from build123d import *

# Parameters (mm, degrees)
SKETCH_1_W          = 50
SKETCH_1_H          = 22
SKETCH_1_R          = 1.05
EXTRUDE_1_DEPTH     = 2
SKETCH_2_W          = 25
SKETCH_2_H          = 2
EXTRUDE_2_DEPTH     = 20
SKETCH_3_R          = 1.65
CUT_EXTRUDE_1_DEPTH = 30
SKETCH_4_W          = 35
SKETCH_4_H          = 15
CUT_EXTRUDE_2_DEPTH = 30


with BuildPart() as part:
    # 草图1 → 凸台-拉伸1 (new body)
    with BuildSketch(Plane(origin=(0, 0, 0), x_dir=(1, 0, 0), z_dir=(0, 1, 0))):
        Rectangle(SKETCH_1_W, SKETCH_1_H)
        with Locations(Location((-21.41, 8.87, 0), (0, 0, 270))):
            Circle(SKETCH_1_R, mode=Mode.SUBTRACT)
        with Locations(Location((-21.41, -8.87, 0), (0, 0, 90))):
            Circle(SKETCH_1_R, mode=Mode.SUBTRACT)
        with Locations(Location((21.41, -8.87, 0), (0, 0, 270))):
            Circle(SKETCH_1_R, mode=Mode.SUBTRACT)
        with Locations(Location((21.41, 8.87, 0), (0, 0, 90))):
            Circle(SKETCH_1_R, mode=Mode.SUBTRACT)
    extrude(amount=EXTRUDE_1_DEPTH)

    # 草图2 → 凸台-拉伸2 (add)
    with BuildSketch(Plane(origin=(0, 2, 0), x_dir=(1, 0, 0), z_dir=(0, 1, 0))):
        Rectangle(SKETCH_2_W, SKETCH_2_H)
    extrude(amount=EXTRUDE_2_DEPTH)

    # 草图3 → 切除-拉伸1 (cut)
    with BuildSketch(Plane.XY.offset(1)):
        with Locations((-5, 22)):
            Circle(SKETCH_3_R)
        with Locations((-5, 12)):
            Circle(SKETCH_3_R)
        with Locations((5, 12)):
            Circle(SKETCH_3_R)
        with Locations((5, 22)):
            Circle(SKETCH_3_R)
    extrude(amount=-CUT_EXTRUDE_1_DEPTH, mode=Mode.SUBTRACT)

    # 草图4 → 切除-拉伸2 (cut)
    with BuildSketch(Plane(origin=(0, 2, 0), x_dir=(1, 0, 0), z_dir=(0, 1, 0))):
        with Locations((0, -11)):
            Rectangle(SKETCH_4_W, SKETCH_4_H)
        with Locations((0, 11)):
            Rectangle(SKETCH_4_W, SKETCH_4_H)
    extrude(amount=-CUT_EXTRUDE_2_DEPTH, mode=Mode.SUBTRACT)


solid = part.part
Work out the finished part from the listing and answer in its coordinate system (mm). A direction names the side the tool comes from. Give positions to 0.01 mm unless a question says otherwise; leave off trailing zeros. Order: outer loops, then holes, each group sorted by start corner. A loop starts at its lowest first (then second) coordinate and runs counter-clockwise, first axis right, second up. Notation, with made-up numbers: (40.25, 28) - (94.25, 28) arc R25 ccw to (94.25, 51) - close; hole circle Ø11 at (-4, -38.75). An arc over 180 degrees is marked (long way). Answer as CSV lines item,"result". Start each with the question number.
Q1. Find the intervals of material crossed by L1, parallel to X at y = 0.95, z = -8.87; L2, parallel to Y at x = -5, z = -0.15; L3, parallel to Z at x = 1.5, y = 21.25, in increasing order. Write a range as [from, to].
Q2. The mould has two halves that part along Y. Classify faces 4 (the face through (-6.31, 11, 0.01)), 5 (the face through (10, 22, 0)), 6 (the face through (-25, 1, 0)): +Y half, -Y half, draft (parallel to the pull), parting line (faces both ways), or undercut.
Q3. For faces 1 (the face through (-17.5, 1, -7)), 2 (the face through (-17.5, 1, 7)), 3 (the face through (0, 12, 1)), determine the directions among +Z, -Z, +X, -X, +Y, -Y from which every point of the face is accessible in a straight line to the end or side of a thin tool.
Q4. The part is cut by section D-D (y = 1.5). Write down the section's boundary in (x, z).
Q5. The part is cut by section A-A (z = -8.87). Write down the section's boundary in (x, y), then the cut area to 3 significant figures.
Q6. The part is cut by section B-B (y = 12). Write down the section's boundary in (x, z), then the cut area to 3 significant figures.
Q7. Given pin 1 Ø3 at (x, y) = (9, 4.5) entering from -Z; pin 2 Ø8 at (x, y) = (-3, 18.5) entering from +Z; pin 3 Ø3 at (y, z) = (16, 1) entering from +X, each flat-ended and moving along its own axis, determine where each tip first touches the part or whether it passes through.
Q8. The part is cut by section C-C (x = 21.41). Write down the section's boundary in (y, z), then the cut area to 3 significant figures.
Check result:
1,L1,"x = [-25, -22.46], [-20.36, -17.5], [17.5, 20.36], [22.46, 25]"
1,L2,"y = [0, 10.35], [13.65, 20.35]"
1,L3,"z = [-1, 1]"
2,face 4,"undercut"
2,face 5,"+Y half"
2,face 6,"draft"
3,face 1,"-Z, +Y, -Y"
3,face 2,"+Z, +Y, -Y"
3,face 3,"+Z, +X, -X, +Y"
4,outline,"(-25, -11) - (-17.5, -11) - (-17.5, -3.5) - (17.5, -3.5) - (17.5, -11) - (25, -11) - (25, 11) - (17.5, 11) - (17.5, 3.5) - (-17.5, 3.5) - (-17.5, 11) - (-25, 11) - close; hole circle Ø2.1 at (-21.41, -8.87); hole circle Ø2.1 at (-21.41, 8.87); hole circle Ø2.1 at (21.41, -8.87); hole circle Ø2.1 at (21.41, 8.87)"
5,outline,"(-25, 0) - (-22.46, 0) - (-22.46, 2) - (-25, 2) - close; (-20.36, 0) - (-17.5, 0) - (-17.5, 2) - (-20.36, 2) - close; (17.5, 0) - (20.36, 0) - (20.36, 2) - (17.5, 2) - close; (22.46, 0) - (25, 0) - (25, 2) - (22.46, 2) - close"
5,area,"21.6 mm²"
6,outline,"(-12.5, -1) - (-6.65, -1) - (-6.65, 1) - (-12.5, 1) - close; (-3.35, -1) - (3.35, -1) - (3.35, 1) - (-3.35, 1) - close; (6.65, -1) - (12.5, -1) - (12.5, 1) - (6.65, 1) - close"
6,area,"36.8 mm²"
7,pin 1,"stops at z = -1"
7,pin 2,"stops at z = 1"
7,pin 3,"stops at x = 12.5"
8,outline,"(0, -11) - (2, -11) - (2, -9.92) - (0, -9.92) - close; (0, -7.82) - (2, -7.82) - (2, 7.82) - (0, 7.82) - close; (0, 9.92) - (2, 9.92) - (2, 11) - (0, 11) - close"
8,area,"35.6 mm²"
